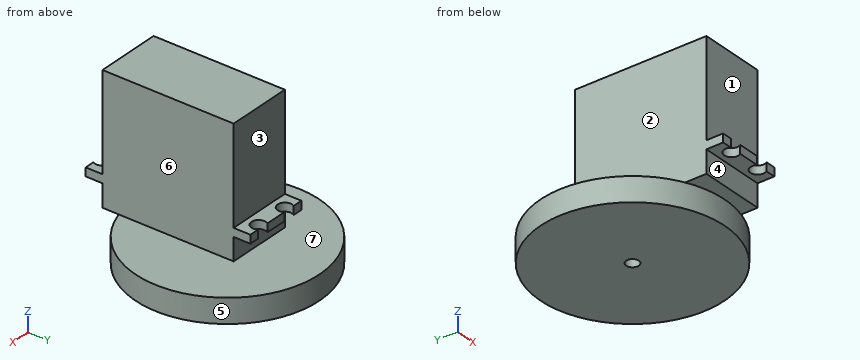
```python
from build123d import *

# Parameters (mm, degrees)
SKETCH1_W           = 19.812
SKETCH1_H           = 39.878
BOSS_EXTRUDE1_DEPTH = 29.21
BOSS_EXTRUDE2_DEPTH = 2.54
SKETCH3_W           = 19.812
SKETCH3_H           = 39.878
BOSS_EXTRUDE3_DEPTH = 6.858
SKETCH4_R           = 6.35
BOSS_EXTRUDE4_DEPTH = 1.524
SKETCH9_R           = 27.94
SKETCH9_R_2         = 1.905
BOSS_EXTRUDE6_DEPTH = 7.366


with BuildPart() as part:
    # Sketch1 → Boss-Extrude1 (new body)
    with BuildSketch(Plane.XY):
        with Locations((9.906, 19.939)):
            Rectangle(SKETCH1_W, SKETCH1_H)
    extrude(amount=BOSS_EXTRUDE1_DEPTH)

    # Sketch2 → Boss-Extrude2 (add)
    with BuildSketch(Plane(origin=(0, 0, 0), x_dir=(-1, 0, 0), z_dir=(0, 0, -1))):
        with BuildLine():
            Line((0, -5.08), (-3.048725862, -5.08))
            ThreePointArc((-3.048725862, -5.08), (-4.826, -1.6256), (-6.603274138, -5.08))
            Line((-6.603274138, -5.08), (-13.208725862, -5.08))
            ThreePointArc((-13.208725862, -5.08), (-14.986, -1.6256), (-16.763274138, -5.08))
            Line((-16.763274138, -5.08), (-19.812, -5.08))
            Line((-19.812, -5.08), (-19.812, 44.958))
            Line((-19.812, 44.958), (-16.763274138, 44.958))
            ThreePointArc((-16.763274138, 44.958), (-14.986, 41.5036), (-13.208725862, 44.958))
            Line((-13.208725862, 44.958), (-6.603274138, 44.958))
            ThreePointArc((-6.603274138, 44.958), (-4.826, 41.5036), (-3.048725862, 44.958))
            Line((-3.048725862, 44.958), (0, 44.958))
            Line((0, 44.958), (0, -5.08))
        make_face()
    extrude(amount=BOSS_EXTRUDE2_DEPTH)

    # Sketch3 → Boss-Extrude3 (add)
    with BuildSketch(Plane(origin=(0, 0, -2.54), x_dir=(-1, 0, 0), z_dir=(0, 0, -1))):
        with Locations((-9.906, 19.939)):
            Rectangle(SKETCH3_W, SKETCH3_H)
    extrude(amount=BOSS_EXTRUDE3_DEPTH)

    # Sketch4 → Boss-Extrude4 (add)
    with BuildSketch(Plane(origin=(0, 0, -9.398), x_dir=(-1, 0, 0), z_dir=(0, 0, -1))):
        with Locations((-9.906, 30.226)):
            Circle(SKETCH4_R)
    extrude(amount=BOSS_EXTRUDE4_DEPTH)

    # Sketch9 → Boss-Extrude6 (add)
    with BuildSketch(Plane(origin=(0, 0, -10.922), x_dir=(-1, 0, 0), z_dir=(0, 0, -1))):
        with Locations((-9.906, 30.226)):
            Circle(SKETCH9_R)
        with Locations((-9.906, 30.226)):
            Circle(SKETCH9_R_2, mode=Mode.SUBTRACT)
    extrude(amount=BOSS_EXTRUDE6_DEPTH)


solid = part.part
```
Verification items for the finished model (mm, model axes). Face numbers are marked on the shaded views. A direction names the side the tool comes from. Round coordinates to 2 decimals unless told otherwise and drop trailing zeros. Order: outer loops, then holes, each group sorted by start corner. A loop starts at its lowest first (then second) coordinate and runs counter-clockwise, first axis right, second up.
1) Cross-section at C-C, the plane y = 33.5. Record the cut outline in (x, z).
Geometry says:
outline: (-17.84, -18.29) - (37.65, -18.29) - (37.65, -10.92) - (15.35, -10.92) - (15.35, -9.4) - (19.81, -9.4) - (19.81, 29.21) - (0, 29.21) - (0, -9.4) - (4.47, -9.4) - (4.47, -10.92) - (-17.84, -10.92) - close
2) Cross-section at B-B, the plane y = 9.5. Record the cut outline in (x, z), plus the area to 3 significant figures.
Geometry says:
outline: (-8.83, -18.29) - (28.64, -18.29) - (28.64, -10.92) - (-8.83, -10.92) - close; (0, -9.4) - (19.81, -9.4) - (19.81, 29.21) - (0, 29.21) - close
area: 1,040 mm2
3) Material ranges on line 1 (X direction, y = -3.81, z = -1.1); line 2 (Z direction, x = 19, y = 14); line 3 (Y direction, x = 18, z = 17.5), recorded low to high.
Geometry says:
line 1: x = 0 to 2.64, 7.01 to 12.8, 17.17 to 19.81
line 2: z = -18.29 to -10.92, -9.4 to 29.21
line 3: y = 0 to 39.88
4) Cross-section at A-A, the plane y = -3.81. Record the cut outline in (x, z).
Geometry says:
outline: (0, -2.54) - (2.64, -2.54) - (2.64, 0) - (0, 0) - close; (7.01, -2.54) - (12.8, -2.54) - (12.8, 0) - (7.01, 0) - close; (17.17, -2.54) - (19.81, -2.54) - (19.81, 0) - (17.17, 0) - close
5) Draft check along X on the marked faces 5, 6 and 7. Enter one of: +X half, -X half, draft (parallel to the pull), parting line (faces both ways), or undercut.
Geometry says:
face 5: parting line
face 6: +X half
face 7: draft
6) Depth check by flat-ended pin: pin 1 (4 mm diameter, centred on x = -5, z = -7.5, fed in from +Y); pin 2 (5.5 mm diameter, centred on x = 8, y = 43, fed in from +Z); pin 3 (22 mm diameter, centred on x = 5.5, z = 10.5, fed in from +Y); pin 4 (10 mm diameter, centred on y = 4, z = -13, fed in from -X). Enter the tip coordinate at first touch or a pass-through.
Geometry says:
pin 1: passes through
pin 2: stops at z = 0
pin 3: stops at y = 44.96
pin 4: stops at x = -8.26
7) Cross-section at D-D, the plane z = -4. Record the cut outline in (x, y), plus the area to 3 significant figures.
Geometry says:
outline: (0, 0) - (19.81, 0) - (19.81, 39.88) - (0, 39.88) - close
area: 790 mm2
8) Tool access check on the marked faces 1, 2, 3 and 4. Record the directions out of +Z, -Z, +X, -X, +Y, -Y that give a thin tool (end or side, any length) a straight path to the whole face; none if there is none.
Geometry says:
face 1: +Z, +X, -X, -Y
face 2: +Z, -X, +Y, -Y
face 3: +Z, +X, -X, +Y
face 4: -Z, +X, -X, -Y
